Read the model definition and answer for the solid it produces. Units are mm, in the model's axes. A direction names the side the tool comes from. Round coordinates to 2 decimals unless told otherwise and drop trailing zeros. Write each loop counter-clockwise with the first axis right and the second up, starting at its lowest first coordinate (ties: lowest second). Pieces come first, ordered by that corner, then holes. Notation, with made-up numbers: (-33.5, 60) - (15.5, 60) arc R20 cw to (15.5, 83) - close; hole circle Ø6 at (-11.5, -35). An arc over 180 degrees is marked (long way). Use one line per item in the form item = value. Start each with the question number.
1) The part is cut by section C-C, the plane z = 6. Give the vertices of the cut face in (x, y) (3 decimals), plus the area to 3 significant figures.
2) The part is cut by section B-B, the plane x = -20.25. Give the vertices of the cut face in (y, z) (3 decimals), plus the area to 3 significant figures.
3) Consider line 1 along Z through (x, y) = (-1.75, 7.5); line 2 along Z through (x, y) = (-7.5, 7.5); line 3 along Z through (x, y) = (-20.75, 6). Determine where each line is inside the solid, lowest interval first. Write a range as from..to.
4) Each of these flat-tipped pins is pushed along its axis until it touches: pin 1 (3.5 mm diameter, centred on x = -1.67, y = 4.76, fed in from -Z); pin 2 (4.5 mm diameter, centred on x = -1.67, y = 4.76, fed in from -Z). Where does it stop, or does it pass through?
5) The part is cut by section A-A, the plane z = -14. Give the vertices of the cut face in (x, y) (1 decimal), plus the area to 3 significant figures.
6) For a pull along Z with two mould halves and no side action, classify faces 4 (the face through (-1.548, 5.067, 3.637)), 5 (the face through (0.57, 4.7, 6.41)), 6 (the face through (1.501, 5, -13)) as released by +Z, released by -Z, zero draft, split by the parting line, or undercut.
7) The part is cut by section D-D, the plane x = -7.5. Give the vertices of the cut face in (y, z) (3 decimals).
8) For faces 1 (the face through (-2.958, 3.363, -2.971)), 2 (the face through (-14, 0, -9)), 3 (the face through (-4, 5, -8.481)), determine the directions among +Z, -Z, +X, -X, +Y, -Y from which every point of the face is accessible in a straight line to the end or side of a thin tool.
from build123d import *

# Parameters (mm, degrees)
BOSS_EXTRUDE1_DEPTH        = 9.525
F_8_CLEARANCE_HOLE1_D      = 4.4958
F_10_CLEARANCE_HOLE1_D     = 5.1054
F_10_CLEARANCE_HOLE1_DEPTH = 6.35


with BuildPart() as part:
    # Sketch1 → Boss-Extrude1 (new body)
    with BuildSketch(Plane(origin=(0, 0, 0), x_dir=(1, 0, 0), z_dir=(0, 1, 0))):
        with BuildLine():
            Line((1.500621967, 8.481252019), (1.500621967, -9.679747981))
            Line((1.500621967, -9.679747981), (-23.899378033, -9.679747981))
            Line((-23.899378033, -9.679747981), (-23.899378033, 15.720252019))
            Line((-23.899378033, 15.720252019), (1.500621967, 15.720252019))
            Line((1.500621967, 15.720252019), (1.500621967, 9.370252019))
            Line((1.500621967, 9.370252019), (-11.199378033, 9.370252019))
            ThreePointArc((-11.199378033, 9.370252019), (-12.879430115, -3.103466214), (-7.959010924, 8.481252019))
            Line((-7.959010924, 8.481252019), (1.500621967, 8.481252019))
        make_face()
    extrude(amount=BOSS_EXTRUDE1_DEPTH)

    # #8 Clearance Hole1 (through all)
    with Locations(Plane(origin=(0, 9.525, 0), x_dir=(1, 0, 0), z_dir=(0, 1, 0))):
        with Locations((-20.724378033, 12.545252019), (-1.674378033, -6.504747981)):
            Hole(F_8_CLEARANCE_HOLE1_D / 2)

    # Sketch4 → #10-24 Tapped Hole1 (revolve, cut)
    with BuildSketch(Plane(origin=(-1.674378033, 4.7625, -8.481252019), x_dir=(0, 1, 0), z_dir=(1, 0, 0))):
        Polygon((0, 0), (0, 12.316824014), (1.89865, 11.176), (1.89865, 0), align=None)
    revolve(axis=Axis((-1.674378033, 4.7625, -14.831252019), (0, 0, 1)), mode=Mode.SUBTRACT)

    # #10 Clearance Hole1
    with Locations(Plane(origin=(0, 0, -15.720252019), x_dir=(-1, 0, 0), z_dir=(0, 0, -1))):
        with Locations((1.674378033, 4.7625)):
            Hole(F_10_CLEARANCE_HOLE1_D / 2, depth=F_10_CLEARANCE_HOLE1_DEPTH)


solid = part.part
Geometry results:
q1.outline = (-23.899, 0) - (-3.865, 0) - (-3.865, 9.525) - (-23.899, 9.525) - close; (0.516, 0) - (1.501, 0) - (1.501, 9.525) - (0.516, 9.525) - close
q1.area = 200 mm2
q2.outline = (0, -15.72) - (9.525, -15.72) - (9.525, -14.743) - (0, -14.743) - close; (0, -10.348) - (9.525, -10.348) - (9.525, 9.68) - (0, 9.68) - close
q2.area = 200 mm2
q3.line_1 = -15.72..-9.37, -8.48..4.26, 8.75..9.68
q3.line_2 = -15.72..-9.37, -8.48..-8.18, 2.14..9.68
q3.line_3 = -15.72..-14.79, -10.3..9.68
q4.pin_1 = 2.78
q4.pin_2 = -8.48
q5.outline = (-23.9, 0) - (-22.4, 0) - (-22.4, 9.5) - (-23.9, 9.5) - close; (-19, 0) - (1.5, 0) - (1.5, 9.5) - (-19, 9.5) - close; hole circle Ø5.1 at (-1.7, 4.8)
q5.area = 189 mm2
q6.face_4 = released by -Z
q6.face_5 = undercut
q6.face_6 = zero draft
q7.outline = (0, -15.72) - (9.525, -15.72) - (9.525, -9.37) - (0, -9.37) - close; (0, -8.481) - (9.525, -8.481) - (9.525, -8.181) - (0, -8.181) - close; (0, 2.141) - (9.525, 2.141) - (9.525, 9.68) - (0, 9.68) - close
q8.face_1 = -Z
q8.face_2 = +Z, -Z, +X, -X, -Y
q8.face_3 = +X, +Y, -Y
